Check sheet for the modelled part. Datum: model origin and axes. Units: mm. Round coordinates to 2 decimals unless told otherwise and drop trailing zeros. Order: outer loops, then holes, each group sorted by start corner. A loop starts at its lowest first (then second) coordinate and runs counter-clockwise, first axis right, second up. Notation, with made-up numbers: (-31.75, 88.25) -> (-7.75, 88.25) arc R22 cw to (-7.75, 125.25) -> close; hole circle Ø9 at (-27, -9). An arc over 180 degrees is marked (long way). Answer in a Markdown table with one row per item. Add a question column.
1. Sectioned sample at B-B, the plane y = 0.5. Record the boundary of the cut face in (x, z), then the cut area to 3 significant figures.
2. Sectioned sample at A-A, the plane z = 4.5. Record the boundary of the cut face in (x, y), then the cut area to 3 significant figures.
3. Depth check by flat-ended pin: P1, Ø2, axis at x = 46.5, z = 14.5, coming from the +Y side; P2, Ø5, axis at x = 37.5, y = 5.43, coming from the +Z side; P3, Ø5, axis at x = 29.5, z = 9.57, coming from the +Y side; P4, Ø10, axis at y = 9, z = 10, coming from the +X side. Enter the tip coordinate at first touch or a pass-through.
4. Draft check along X on faces 1 (the cylindrical face through (59.217, -1.872, 9.437)), 2 (the conical face through (20.613, -3.419, -0.287)), 3 (the cylindrical face through (33.536, 5.95, 10.443)). Enter one of: +X half, -X half, draft (parallel to the pull), parting line (faces both ways), or undercut.
5. Material ranges on L1, parallel to X at y = 6.5, z = 11.5; L2, parallel to X at y = 5.25, z = 3.5; L3, parallel to X at y = 9.5, z = 8.5, recorded low to high. Write a range as from..to.
6. Sectioned sample at C-C, the plane y = 5. Count the separate pieces of the cut face and the enclosed holes in it, then the cut area to 3 significant figures.
```python
from build123d import *

# Parameters (mm, degrees)
SKETCH1_W                      = 40
SKETCH1_H                      = 20
BOSS_EXTRUDE1_DEPTH            = 17
SKETCH2_W                      = 15
SKETCH2_H                      = 14
CUT_EXTRUDE1_DEPTH             = 21
F_4_4_4_4_DIAMETER_HOLE1_D     = 4.4
F_4_4_4_4_DIAMETER_HOLE1_DEPTH = 17
F_4_2_4_2_DIAMETER_HOLE1_D     = 4.2
F_4_2_4_2_DIAMETER_HOLE1_DEPTH = 17
FILLET1_R                      = 1
FILLET2_R                      = 3
FILLET3_R                      = 7
CHAMFER1_SIZE                  = 0.5


with BuildPart() as part:
    # Sketch1 → Boss-Extrude1 (new body)
    with BuildSketch(Plane.XZ.offset(4.571066784)):
        with Locations((39.501752658, 9.570440181)):
            Rectangle(SKETCH1_W, SKETCH1_H)
    extrude(amount=-BOSS_EXTRUDE1_DEPTH)

    # Sketch2 → Cut-Extrude1 (cut, through all)
    with BuildSketch(Plane.XY.offset(19.570440181)):
        with Locations((52.001752658, 5.428933216)):
            Rectangle(SKETCH2_W, SKETCH2_H)
    extrude(amount=-CUT_EXTRUDE1_DEPTH, mode=Mode.SUBTRACT)

    # Ø4.4 (4.4) Diameter Hole1
    with Locations(Plane(origin=(0, -4.571066784, 0), x_dir=(-1, 0, 0), z_dir=(0, -1, 0))):
        with Locations((-51.501752658, -9.570440181)):
            Hole(F_4_4_4_4_DIAMETER_HOLE1_D / 2, depth=F_4_4_4_4_DIAMETER_HOLE1_DEPTH)

    # Ø4.2 (4.2) Diameter Hole1
    with Locations(Plane(origin=(0, 12.428933216, 0), x_dir=(1, 0, 0), z_dir=(0, 1, 0))):
        with Locations((29.501752658, -9.570440181)):
            Hole(F_4_2_4_2_DIAMETER_HOLE1_D / 2, depth=F_4_2_4_2_DIAMETER_HOLE1_DEPTH)

    # Sketch7 → Hole1 (revolve, cut)
    with BuildSketch(Plane(origin=(37.501752658, 5.428933216, 19.570440181), x_dir=(0, -1, 0), z_dir=(1, 0, 0))):
        Polygon((0, 0), (0, 20), (3, 20), (3, 19), (4, 18), (4, 0), align=None)
    revolve(axis=Axis((37.501752658, 5.428933216, 25.70046408), (0, 0, -1)), mode=Mode.SUBTRACT)

    # Fillet1
    fillet1_edges = [part.edges().sort_by_distance(p)[0] for p in [
        (59.501752658, -1.571066784, 9.570440181),
        (44.501752658, -1.571066784, 9.570440181),
        (59.501752658, -4.571066784, 9.570440181),
    ]]
    fillet(fillet1_edges, radius=FILLET1_R)

    # Fillet2
    fillet2_edges = [part.edges().sort_by_distance(p)[0] for p in [
        (19.501752658, 12.428933216, 9.570440181),
        (19.501752658, -4.571066784, 9.570440181),
    ]]
    fillet(fillet2_edges, radius=FILLET2_R)

    # Fillet3
    fillet3_edges = [part.edges().sort_by_distance(p)[0] for p in [
        (44.501752658, 12.428933216, 9.570440181),
    ]]
    fillet(fillet3_edges, radius=FILLET3_R)

    # Chamfer1
    chamfer1_edges = [part.edges().sort_by_distance(p)[0] for p in [
        (31.601752658, 12.428933216, 9.570440181),
        (31.601752658, -4.571066784, 9.570440181),
        (37.501752658, 9.428933216, 19.570440181),
        (52.001752658, -1.571066784, 19.570440181),
        (52.001752658, -1.571066784, -0.429559819),
        (59.501752658, -3.071066784, 19.570440181),
        (59.501752658, -3.071066784, -0.429559819),
        (40.501752658, -4.571066784, 19.570440181),
        (59.208859439, -4.278173565, 19.570440181),
        (59.208859439, -1.863960002, 19.570440181),
        (59.208859439, -4.278173565, -0.429559819),
        (59.208859439, -1.863960002, -0.429559819),
        (44.794645876, -1.278173565, 19.570440181),
        (44.794645876, -1.278173565, -0.429559819),
        (40.501752658, -4.571066784, -0.429559819),
        (19.501752658, 3.928933216, -0.429559819),
        (30.001752658, 12.428933216, -0.429559819),
        (20.380432314, 11.55025356, -0.429559819),
        (20.380432314, -3.692387127, -0.429559819),
        (19.501752658, 3.928933216, 19.570440181),
        (20.380432314, 11.55025356, 19.570440181),
        (20.380432314, -3.692387127, 19.570440181),
        (44.501752658, 2.428933216, 19.570440181),
        (44.501752658, 2.428933216, -0.429559819),
        (30.001752658, 12.428933216, 19.570440181),
        (42.451500126, 10.378680685, 19.570440181),
        (42.451500126, 10.378680685, -0.429559819),
    ]]
    chamfer(chamfer1_edges, length=CHAMFER1_SIZE)


solid = part.part
```
Answer key:
| question | item | result |
|---|---|---|
| 1 | outline | (19.5, 0.07) -> (20, -0.43) -> (44, -0.43) -> (44.5, 0.07) -> (44.5, 19.07) -> (44, 19.57) -> (20, 19.57) -> (19.5, 19.07) -> close; hole circle Ø4.2 at (29.5, 9.57) |
| 1 | area | 486 mm² |
| 2 | outline | (19.5, -1.57) arc R3 ccw to (22.5, -4.57) -> (58.5, -4.57) arc R1 ccw to (59.5, -3.57) -> (59.5, -2.57) arc R1 ccw to (58.5, -1.57) -> (45.5, -1.57) arc R1 cw to (44.5, -0.57) -> (44.5, 5.43) arc R7 ccw to (37.5, 12.43) -> (22.5, 12.43) arc R3 ccw to (19.5, 9.43) -> close; hole circle Ø8 at (37.5, 5.43) |
| 2 | area | 405 mm² |
| 3 | P1 | stops at y = -1.57 |
| 3 | P2 | passes through |
| 3 | P3 | stops at y = 12.33 |
| 3 | P4 | stops at x = 44.5 |
| 4 | face 1 | +X half |
| 4 | face 2 | -X half |
| 4 | face 3 | undercut |
| 5 | L1 | x = 19.5..28.67, 30.33..33.65, 41.36..44.42 |
| 5 | L2 | x = 19.5..33.51, 41.5..44.5 |
| 5 | L3 | x = 19.5..27.7, 31.31..43.2 |
| 6 | separate pieces | 2 |
| 6 | enclosed holes | 1 |
| 6 | area | 329 mm² |
